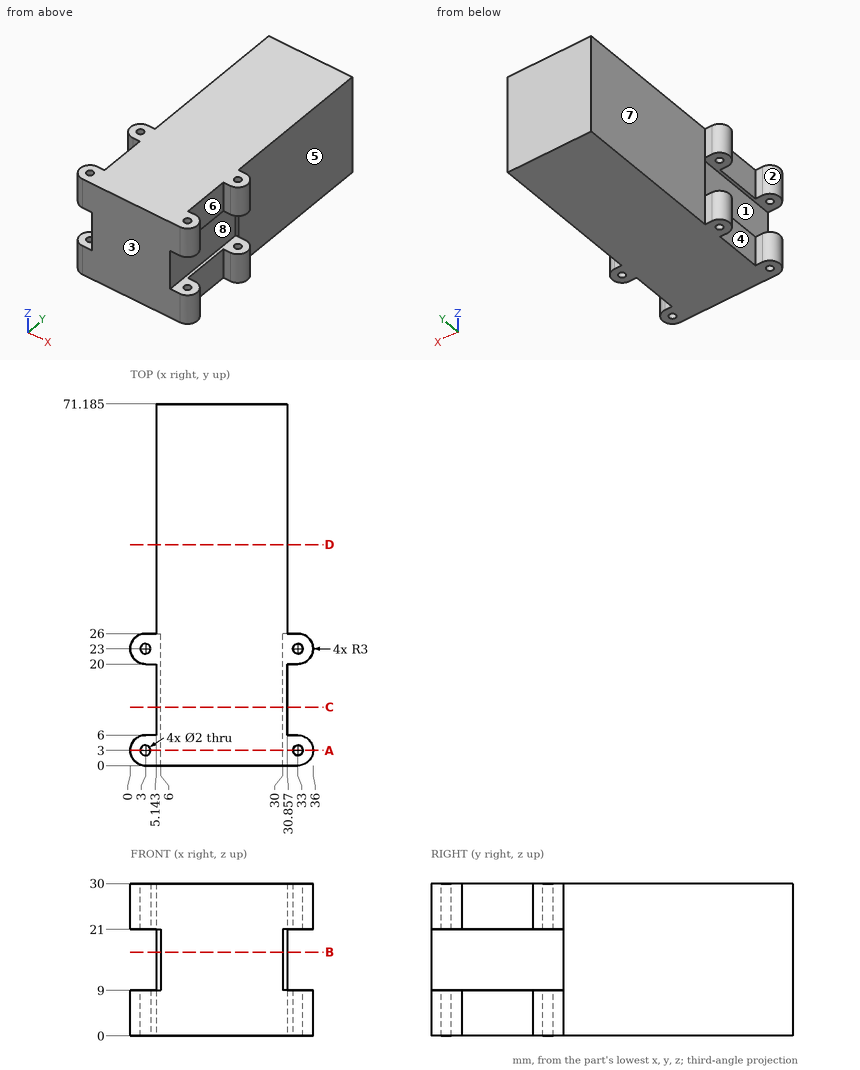
The drawing under review shows one solid part. Ordinate dimensions are in mm from its lowest x, y, z. A direction names the side the tool comes from. Round coordinates to 2 decimals unless told otherwise and drop trailing zeros. Write each loop counter-clockwise with the first axis right and the second up, starting at its lowest first coordinate (ties: lowest second). Pieces come first, ordered by that corner, then holes. Notation, with made-up numbers: (35, -27.75) -> (57, -27.75) arc R21 ccw to (57, 2.25) -> close; hole circle Ø9 at (-4, 88.5). An arc over 180 degrees is marked (long way). One line per question, with ' | ' between items.
(1) Take a section at C-C, the plane y = 11.5. State the section outline as (x, z) points.
Result sheet:
outline: (5.14, 0) -> (30.86, 0) -> (30.86, 9) -> (30, 9) -> (30, 21) -> (30.86, 21) -> (30.86, 30) -> (5.14, 30) -> (5.14, 21) -> (6, 21) -> (6, 9) -> (5.14, 9) -> close
(2) Draft analysis for pull direction Y (two halves, no side actions). For the marked faces 1, 2 and 3, state which applies: released by +Y, released by -Y, zero draft, split by the parting line, or undercut.
Result sheet:
face 1: zero draft | face 2: undercut | face 3: released by -Y
(3) Insertion check: P1, Ø5, axis at x = 34.5, y = 11.5, coming from the +Z side; P2, Ø0.7, axis at x = 30.5, z = 13.5, coming from the -Y side; P3, Ø1.1, axis at x = 32.5, z = 3, coming from the +Y side; P4, Ø5, axis at y = 43, z = 16.5, coming from the +X side. Each pin has a flat end and moves straight along its axis. Give the tip position at first contact, or say it passes through.
Result sheet:
P1: through | P2: y = 26 | P3: y = 26 | P4: x = 30.86
(4) Take a section at A-A, the plane y = 3. State the section outline as (x, z) points.
Result sheet:
outline: (0, 0) -> (2, 0) -> (2, 9) -> (0, 9) -> close; (0, 21) -> (2, 21) -> (2, 30) -> (0, 30) -> close; (4, 0) -> (32, 0) -> (32, 9) -> (30, 9) -> (30, 21) -> (32, 21) -> (32, 30) -> (4, 30) -> (4, 21) -> (6, 21) -> (6, 9) -> (4, 9) -> close; (34, 0) -> (36, 0) -> (36, 9) -> (34, 9) -> close; (34, 21) -> (36, 21) -> (36, 30) -> (34, 30) -> close
(5) Wall thickness on line 1 (Y direction, x = 33, z = 5.5); line 2 (X direction, y = 47, z = 13); line 3 (Y direction, x = 5, z = 23): over which ranges is each line inside the solid? List them lowest first. Write a range as [from, to].
Result sheet:
line 1: [0, 2], [4, 6], [20, 22], [24, 26] | line 2: [5.14, 30.86] | line 3: [0, 6], [20, 26]
(6) Take a section at D-D, the plane y = 43.5. State the section outline as (x, z) points.
Result sheet:
outline: (5.14, 0) -> (30.86, 0) -> (30.86, 30) -> (5.14, 30) -> close
(7) Take a section at B-B, the plane z = 16.5. State the section outline as (x, y) points (1 decimal), and give its area (3 significant figures).
Result sheet:
outline: (5.1, 26) -> (6, 26) -> (6, 0) -> (30, 0) -> (30, 26) -> (30.9, 26) -> (30.9, 71.2) -> (5.1, 71.2) -> close | area: 1,790 mm2
(8) Machinability: for the marked faces 4, 5, 6, 7 and 8, which of the approach directions +Z, -Z, +X, -X, +Y, -Y give a long, thin tool a straight path to every point of the face, cutting with its end or side? Answer none if there is none.
Result sheet:
face 4: +Z, -Z, -X | face 5: +Z, -Z, +X, +Y | face 6: +Z, -Z, +X | face 7: +Z, -Z, -X, +Y | face 8: +X, -Y
